Geometry check sheet. Reference: the model listing, model coordinates, mm. Face numbers are marked on the shaded views. A direction names the side the tool comes from. Round coordinates to 2 decimals unless told otherwise and drop trailing zeros. Loops run counter-clockwise (first coordinate to the right, second up) from the corner with the lowest first, then second, coordinate; pieces in that order, holes last. Notation, with made-up numbers: (-37, 85) - (-25, 85) arc R15 cw to (-25, 104) - close; hole circle Ø6 at (22.5, 15.5). An arc over 180 degrees is marked (long way). Answer in a Markdown table with one row per item. Add a question column.
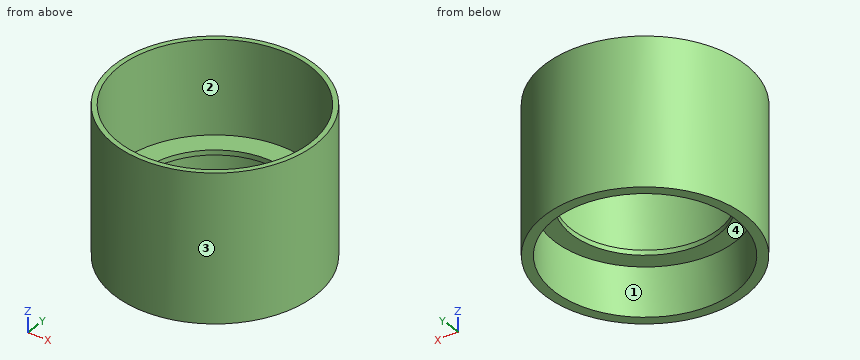
Autodesk Inventor part; units mm, degrees
ref_plane "YZ Plane" through (0, 0, 0) normal (1, 0, 0) x (0, 1, 0)
ref_plane "XZ Plane" through (0, 0, 0) normal (0, 1, 0) x (-1, 0, 0)
ref_plane "XY Plane" through (0, 0, 0) normal (0, 0, 1) x (1, 0, 0)
sketch "Sketch1" plane through (0, 0, 0) normal (0, 0, 1) x (1, 0, 0)
  circle A0 centre (0, 0) radius 20.5
  dimension "d0" = 41
extrude "Extrusion1" add sketch "Sketch1" along normal blind 30
sketch "Sketch2" plane through (0, 0, 0) normal (0, 0, -1) x (-1, 0, 0)
  point P0 (0, 0)
  point P1 (0, 0)
hole "Hole1" at (0, 0, 0) direction (0, 0, 1) diameter 37 depth 10
shell "Shell1" thickness 1 removed faces 1 at (3.5154, 4.1371, 30)
thread "Thread1"
sketch "Sketch4" plane through (0, 0, 10) normal (0, 0, -1) x (-1, 0, 0)
  point P0 (0, 0)
  point P1 (0, 0)
hole "Hole2" at (0, 0, 10) direction (0, 0, 1) diameter 30 depth 30
properties part number "Tutup lampu" material "Aluminum 6061-AHC"
Q1. Cross-section at A-A, the plane x = 0. Enter the section's corners in (y, z), plus the area to 3 significant figures.
Q2. Set-up check for the marked faces 1 and 2: record each of +Z, -Z, +X, -X, +Y, -Y from which the full face is reachable in a straight line by a thin tool's end or side.
Q3. Depth check by flat-ended pin: P1, Ø1.5, axis at y = 13.5, z = 21.5, coming from the -X side; P2, Ø10, axis at x = 3.5, z = 18.5, coming from the -Y side; P3, Ø6, axis at x = -12, y = 14, coming from the +Z side; P4, Ø1, axis at y = -14, z = 26, coming from the +X side. Enter the tip coordinate at first touch or a pass-through.
Q4. Scan lines: line 1 (Y direction, x = 0, z = 4.5); line 2 (Y direction, x = 0, z = 10.5); line 3 (X direction, y = 15, z = 24.25). Record each from-to range of solid material in increasing order. Write a range as from..to.
Q5. Cross-section at D-D, the plane z = 20.5. Enter the section's corners in (x, y).
Q6. Release check for a two-part mould opening along Y. For the marked faces 3 and 4 record: +Y half, -Y half, draft (parallel to the pull), parting line (faces both ways), or undercut.
Q7. Cross-section at C-C, the plane z = 8.75. Enter the section's corners in (x, y), plus the area to 3 significant figures.
Check sheet entries:
| question | item | result |
|---|---|---|
| 1 | outline | (-20.5, 0) - (-18.5, 0) - (-18.5, 10) - (-15, 10) - (-15, 11) - (-19.5, 11) - (-19.5, 30) - (-20.5, 30) - close; (15, 10) - (18.5, 10) - (18.5, 0) - (20.5, 0) - (20.5, 30) - (19.5, 30) - (19.5, 11) - (15, 11) - close |
| 1 | area | 89.0 mm² |
| 2 | face 1 | -Z |
| 2 | face 2 | +Z |
| 3 | P1 | x = -16.05 |
| 3 | P2 | y = -20.5 |
| 3 | P3 | z = 30 |
| 3 | P4 | x = 15.43 |
| 4 | line 1 | -20.5..-18.5, 18.5..20.5 |
| 4 | line 2 | -20.5..-15, 15..20.5 |
| 4 | line 3 | -13.97..-12.46, 12.46..13.97 |
| 5 | outline | circle Ø41 at (0, 0); hole circle Ø39 at (0, 0) |
| 6 | face 3 | parting line |
| 6 | face 4 | undercut |
| 7 | outline | circle Ø41 at (0, 0); hole circle Ø37 at (0, 0) |
| 7 | area | 245 mm² |
